Autodesk Inventor part; units mm, degrees
ref_plane "YZ Plane" through (0, 0, 0) normal (1, 0, 0) x (0, 1, 0)
ref_plane "XZ Plane" through (0, 0, 0) normal (0, 1, 0) x (-1, 0, 0)
ref_plane "XY Plane" through (0, 0, 0) normal (0, 0, 1) x (1, 0, 0)
sketch "Sketch1" plane through (0, 0, 0) normal (0, 0, 1) x (1, 0, 0)
  circle A0 centre (0, 0) radius 88
  circle A1 centre (0, 0) radius 138
  line L0 (97.5807, -97.5807) -> (-97.5807, 97.5807) construction
  line L1 (-97.5807, -97.5807) -> (97.5807, 97.5807) construction
  point P0 (0, 88)
  dimension "d44" = 176
  dimension "d23" = 276
extrude "Plate1" add sketch "Sketch1" along normal blind 4
sketch "Sketch6" plane through (0, 0, 0) normal (0, 0, 1) x (1, 0, 0)
  line L0 (0, 0) -> (0, 120) construction
  circle A0 centre (0, 0) radius 120 construction
  line L1 (0, 0) -> (84.8528, 84.8528) construction
  circle A1 centre (84.8528, 84.8528) radius 9
  dimension "d32" = 18
  dimension "d33" = 240
  dimension "d34" = 45
extrude "Cut2" cut sketch "Sketch6" along normal blind 4
pattern_circular "Circular Pattern2" count 8 over 360 about axis through (0, 0, -10) along (0, 0, -1) of "Cut2"
equation "\"d32\" = Flange_d_hole_diam"
equation "\"d33\" = Flange_D1_hole_center"
equation "\"d35\" = Thickness"
equation "\"d2\" = Thickness"
equation "\"BendReliefWidth\" = Thickness"
equation "\"BendReliefDepth\" = 0.5 * Thickness"
equation "\"CornerReliefSize\" = 4 * Thickness"
equation "\"MinimumRemnant\" = 2 * Thickness"
equation "\"TransitionRadius\" = BendRadius"
equation "\"JacobiRadiusSize\" = BendRadius"
equation "\"GapSize\" = Thickness"
equation "\"Octaeder_side\" = d41"
equation "\"Octaeder_flange_lenth\" = d42"
properties part number "DSB 113 drain system loose flange double" material "Stainless Steel"
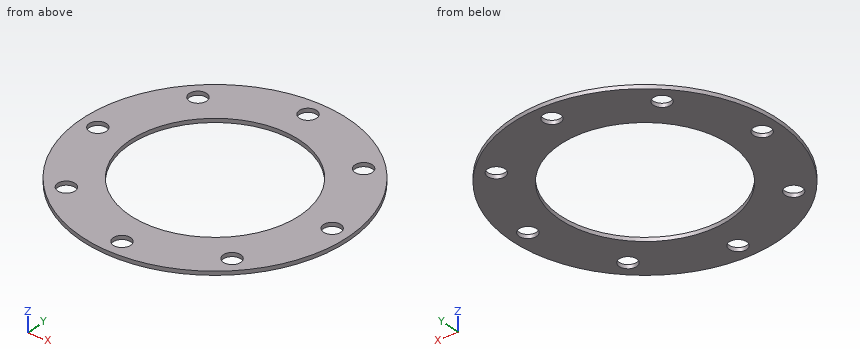
Here's how the part is built. I have some questions about the finished solid (model axes, mm). Round coordinates to 2 decimals unless told otherwise and drop trailing zeros. Order: outer loops, then holes, each group sorted by start corner. A loop starts at its lowest first (then second) coordinate and runs counter-clockwise, first axis right, second up. Notation, with made-up numbers: (9.5, -18) -> (43.5, -18) arc R26 ccw to (43.5, 20) -> close; hole circle Ø6 at (62, 15). An arc over 180 degrees is marked (long way). Use a Markdown table: item, result. Add a question column.
(1) Suppose I cut it at D-D, the plane z = 0.6. Count the separate pieces of the cut face and the enclosed holes in it, and give its area (3 significant figures).
(2) Suppose I cut it at A-A, the plane x = 0. Please give me the cut outline in (y, z), and give its area (3 significant figures).
(3) Suppose I cut it at C-C, the plane y = -35.5. Please give me the cut outline in (x, z), and give its area (3 significant figures).
(4) I need wall thicknesses on line 1 along Y through (x, z) = (0, 2.25); line 2 along Y through (x, z) = (8, 2); line 3 along X through (y, z) = (-64.5, 1.9). Which ranges of each line are inside material? Lowest first, please.
(5) For pin 1 Ø1.5 at (x, z) = (-96.5, 3.5) entering from -Y, with a flat end and sliding along its axis, tell me the tip position at first contact or that it passes through.
Verdict:
| question | item | result |
|---|---|---|
| 1 | separate pieces | 1 |
| 1 | enclosed holes | 9 |
| 1 | area | 33,500 mm2 |
| 2 | outline | (-138, 0) -> (-129, 0) -> (-129, 4) -> (-138, 4) -> close; (-111, 0) -> (-88, 0) -> (-88, 4) -> (-111, 4) -> close; (88, 0) -> (111, 0) -> (111, 4) -> (88, 4) -> close; (129, 0) -> (138, 0) -> (138, 4) -> (129, 4) -> close |
| 2 | area | 256 mm2 |
| 3 | outline | (-133.36, 0) -> (-80.52, 0) -> (-80.52, 4) -> (-133.36, 4) -> close; (80.52, 0) -> (133.36, 0) -> (133.36, 4) -> (80.52, 4) -> close |
| 3 | area | 423 mm2 |
| 4 | line 1 | -138 to -129, -111 to -88, 88 to 111, 129 to 138 |
| 4 | line 2 | -137.77 to -124.12, -115.88 to -87.64, 87.64 to 115.88, 124.12 to 137.77 |
| 4 | line 3 | -122 to -59.86, 59.86 to 122 |
| 5 | pin 1 | y = -99.38 |
